from build123d import *

# Parameters (mm, degrees)
F0_R           = 8.75
F1_DEPTH       = 25
F1_DEPTH_BACK  = 25
F2_R           = 6.75
F3_DEPTH       = 20
F3_DEPTH_BACK  = 20
F4_W           = 18.8391190022
F4_H           = 6.4964373596
F5_DEPTH       = 25.001
F5_DEPTH_BACK  = 25
F6_W           = 10.9675412329
F6_H           = 2.9768612129
F7_DEPTH       = 50
F8_R           = 5
F9_R           = 1.6
F10_DEPTH      = 25.001
F10_DEPTH_BACK = 25.001


with BuildPart() as f1:
    # F0 (on Front) → F1 (new body, two sides)
    with BuildSketch(Plane.XZ) as f1_sk:
        Circle(F0_R)
    extrude(amount=F1_DEPTH)
    extrude(f1_sk.sketch, amount=-F1_DEPTH_BACK)

    # F2 (on Front) → F3 (cut, two sides)
    with BuildSketch(Plane.XZ) as f3_sk:
        Circle(F2_R)
    extrude(amount=-F3_DEPTH, mode=Mode.SUBTRACT)
    extrude(f3_sk.sketch, amount=F3_DEPTH_BACK, mode=Mode.SUBTRACT)

    # F4 (on Front) → F5 (cut, two sides)
    with BuildSketch(Plane.XZ) as f5_sk:
        with Locations((0.2108290792, 5.8920474257)):
            Rectangle(F4_W, F4_H)
    extrude(amount=-F5_DEPTH, mode=Mode.SUBTRACT)
    extrude(f5_sk.sketch, amount=F5_DEPTH_BACK, mode=Mode.SUBTRACT)

    # F6 (on face) → F7 (join, through all)
    with BuildSketch(Plane.XZ.offset(25)):
        with Locations((0, -8.3068438988)):
            Rectangle(F6_W, F6_H)
    extrude(amount=-F7_DEPTH)

    # F8
    f8_edges = [f1.edges().sort_by_distance(p)[0] for p in [
        (5.483771, 0, -6.818413),
        (-5.483771, 0, -6.818413),
    ]]
    fillet(f8_edges, radius=F8_R)

    # F9 (on Front) → F10 (cut, two sides)
    with BuildSketch(Plane.XZ) as f10_sk:
        Circle(F9_R)
    extrude(amount=-F10_DEPTH, mode=Mode.SUBTRACT)
    extrude(f10_sk.sketch, amount=F10_DEPTH_BACK, mode=Mode.SUBTRACT)


solid = f1.part
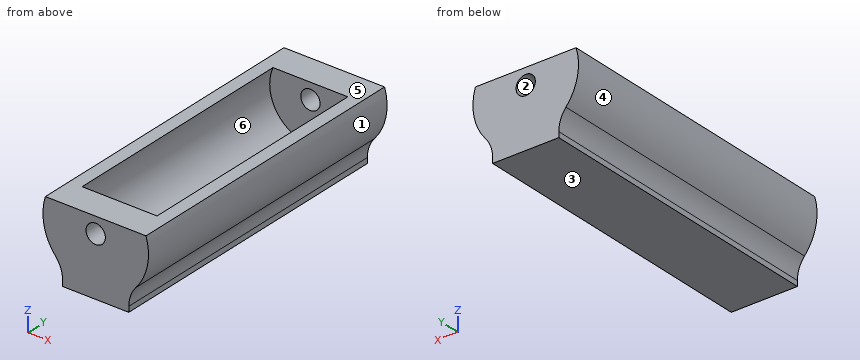
Input: part model. Units: mm. Frame: model coordinates. Face numbers are marked on the shaded views. A direction names the side the tool comes from. Coordinates: 2 decimals unless noted, no trailing zeros. Write each loop counter-clockwise with the first axis right and the second up, starting at its lowest first coordinate (ties: lowest second). Pieces come first, ordered by that corner, then holes. Notation, with made-up numbers: M 87.25,9.5 L 123.25,9.5 A15 ccw 123.25,22.5 Z; hole C -39,25.25 d3. An arc over 180 degrees is marked long. Answer as a JSON object with one key per item and string values. Group by question number.
(1) Section C-C on z = -6.25. Output: boundary loops of the cut face in (x, y).
(2) Ray query, line 1 along Z through (x, y) = (0, 23.2); line 2 along X through (y, z) = (-3, 0); line 3 along Y through (x, z) = (2.5, -1.75). Return the intervals inside material, ascending. Write a range as [from, to].
(3) Contact query for flat-ended pins moving along their axis: P1, Ø3, axis at x = 3.5, y = 7, coming from the +Z side; P2, Ø2, axis at y = -12.5, z = -5, coming from the +X side; P3, Ø5, axis at x = -0.5, y = -14.5, coming from the +Z side. Output: stop coordinate, or through.
(4) Section A-A on x = 0. Output: boundary loops of the cut face in (y, z).
(5) Section D-D on x = -4.5. Output: boundary loops of the cut face in (y, z).
(6) Section B-B on z = 0. Output: boundary loops of the cut face in (x, y).
(7) Mould query, pull axis X, two halves, no side actions, for the marked faces 1, 2, 3 and 4. Classes: pulls with the +X half, pulls with the -X half, needs draft (parallel to the pull), parting line crosses it, or undercut.
(8) Set-up query: the marked faces 5 and 6. Return all of +Z, -Z, +X, -X, +Y, -Y with unobstructed straight access to the full face (end or side cutting, diameter ignored); none if empty.
Result set:
{
 "1": {"outline": "M -6.24,-25 L 6.24,-25 L 6.24,25 L -6.24,25 Z; hole M -2.55,-20 L 2.55,-20 L 2.55,20 L -2.55,20 Z"},
 "2": {"line 1": "z = [-9.8, -1.6], [1.6, 2.64]", "line 2": "x = [-8.75, -6.75], [6.75, 8.75]", "line 3": "y = [-25, -20], [20, 25]"},
 "3": {"P1": "stops at z = -4.53", "P2": "stops at x = 7.78", "P3": "stops at z = -6.05"},
 "4": {"outline": "M -25,-9.8 L 25,-9.8 L 25,-1.6 L 20,-1.6 L 20,-6.75 L -20,-6.75 L -20,-1.6 L -25,-1.6 Z; M -25,1.6 L -20,1.6 L -20,2.64 L -25,2.64 Z; M 20,1.6 L 25,1.6 L 25,2.64 L 20,2.64 Z"},
 "5": {"outline": "M -25,-9.8 L 25,-9.8 L 25,2.64 L 20,2.64 L 20,-5.03 L -20,-5.03 L -20,2.64 L -25,2.64 Z"},
 "6": {"outline": "M -8.75,-25 L -1.6,-25 L -1.6,-20 L -6.75,-20 L -6.75,20 L -1.6,20 L -1.6,25 L -8.75,25 Z; M 1.6,-25 L 8.75,-25 L 8.75,25 L 1.6,25 L 1.6,20 L 6.75,20 L 6.75,-20 L 1.6,-20 Z"},
 "7": {"face 1": "pulls with the +X half", "face 2": "undercut", "face 3": "needs draft", "face 4": "pulls with the -X half"},
 "8": {"face 5": "+Z, +X, -X, +Y, -Y", "face 6": "none"}
}
